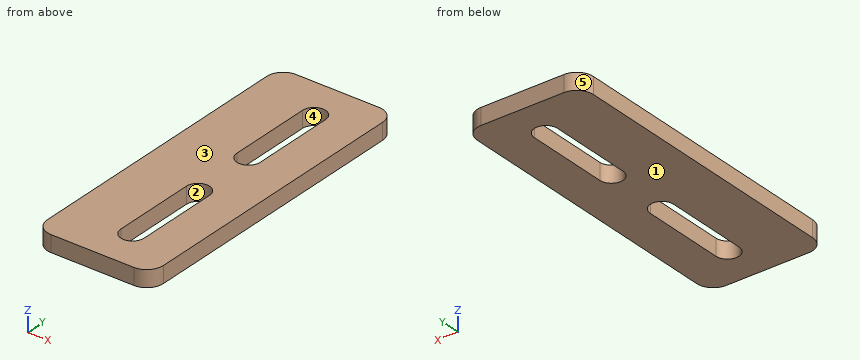
from build123d import *

# Parameters (mm, degrees)
SKETCH1_W           = 35
SKETCH1_H           = 95
BOSS_EXTRUDE1_DEPTH = 5
FILLET1_R           = 5


with BuildPart() as part:
    # Sketch1 → Boss-Extrude1 (new body)
    with BuildSketch(Plane.XY):
        with Locations((17.5, -16.973)):
            Rectangle(SKETCH1_W, SKETCH1_H)
        with BuildLine():
            ThreePointArc((16.5, -7.173), (20, -10.673), (23.5, -7.173))
            Line((23.5, -7.173), (23.5, 18.227))
            ThreePointArc((23.5, 18.227), (20, 21.727), (16.5, 18.227))
            Line((16.5, 18.227), (16.5, -7.173))
        make_face(mode=Mode.SUBTRACT)
        with BuildLine():
            ThreePointArc((23.5, -26.773), (20, -23.273), (16.5, -26.773))
            Line((16.5, -26.773), (16.5, -52.173))
            ThreePointArc((16.5, -52.173), (20, -55.673), (23.5, -52.173))
            Line((23.5, -52.173), (23.5, -26.773))
        make_face(mode=Mode.SUBTRACT)
    extrude(amount=BOSS_EXTRUDE1_DEPTH)

    # Fillet1
    fillet1_edges = [part.edges().sort_by_distance(p)[0] for p in [
        (0, -64.473, 2.5),
        (0, 30.527, 2.5),
        (35, 30.527, 2.5),
        (35, -64.473, 2.5),
    ]]
    fillet(fillet1_edges, radius=FILLET1_R)


solid = part.part
Source: CAD feature listing. Evaluate the final solid. Frame: model axes, mm. Face numbers are marked on the shaded views. A direction names the side the tool comes from. Give positions to 0.01 mm unless a question says otherwise; leave off trailing zeros. Write each loop counter-clockwise with the first axis right and the second up, starting at its lowest first coordinate (ties: lowest second). Pieces come first, ordered by that corner, then holes. Notation, with made-up numbers: (-14, 59) -> (-7, 59) arc R14 ccw to (-7, 66) -> close; hole circle Ø10 at (-7.75, -1.5). An arc over 180 degrees is marked (long way). Write item = value, one per line.
Q1. Reachability of the marked faces 1 and 2 from +Z, -Z, +X, -X, +Y, -Y: full face, straight path, thin tool, end or side. Return the list, or none.
Here are the results:
face_1 = -Z, +X, -X, +Y, -Y
face_2 = +Z, -Z
Q2. Mould query, pull axis X, two halves, no side actions, for the marked faces 3, 4 and 5. Classes: +X half, -X half, draft (parallel to the pull), parting line (faces both ways), or undercut.
Here are the results:
face_3 = draft
face_4 = undercut
face_5 = -X half
Q3. Cut plane B-B on z = 3.95. Return loops of the section in (x, y), then the cut area to 3 significant figures.
Here are the results:
outline = (0, -59.47) arc R5 ccw to (5, -64.47) -> (30, -64.47) arc R5 ccw to (35, -59.47) -> (35, 25.53) arc R5 ccw to (30, 30.53) -> (5, 30.53) arc R5 ccw to (0, 25.53) -> close; hole (16.5, -52.17) arc R3.5 ccw to (23.5, -52.17) -> (23.5, -26.77) arc R3.5 ccw to (16.5, -26.77) -> close; hole (16.5, -7.17) arc R3.5 ccw to (23.5, -7.17) -> (23.5, 18.23) arc R3.5 ccw to (16.5, 18.23) -> close
area = 2,870 mm²
Q4. Line query: line 1 (X direction, y = 9, z = 0.3); line 2 (Y direction, x = 18.5, z = 3.15); line 3 (Y direction, x = 23, z = 2.3). Output: solid intervals per line, ascending. Write a range as from..to.
Here are the results:
line_1 = 0..16.5, 23.5..35
line_2 = -64.47..-55.34, -23.61..-10.34, 21.39..30.53
line_3 = -64.47..-53.98, -24.97..-8.98, 20.03..30.53
Q5. First-contact query: pin 1 (1 mm diameter, centred on x = 4, z = 2, fed in from -Y). Flat tip, straight axial feed; report the tip coordinate or a pass-through.
Here are the results:
pin_1 = -64.45
Q6. Cut plane C-C on x = 20. Return loops of the section in (y, z), then the cut area to 3 significant figures.
Here are the results:
outline = (-64.47, 0) -> (-55.67, 0) -> (-55.67, 5) -> (-64.47, 5) -> close; (-23.27, 0) -> (-10.67, 0) -> (-10.67, 5) -> (-23.27, 5) -> close; (21.73, 0) -> (30.53, 0) -> (30.53, 5) -> (21.73, 5) -> close
area = 151 mm²
Q7. Cut plane A-A on y = -1. Return loops of the section in (x, z), then the cut area to 3 significant figures.
Here are the results:
outline = (0, 0) -> (16.5, 0) -> (16.5, 5) -> (0, 5) -> close; (23.5, 0) -> (35, 0) -> (35, 5) -> (23.5, 5) -> close
area = 140 mm²
